Check sheet for the modelled part. Datum: model origin and axes. Units: mm. Give positions to 0.01 mm unless a question says otherwise; leave off trailing zeros. Loops run counter-clockwise (first coordinate to the right, second up) from the corner with the lowest first, then second, coordinate; pieces in that order, holes last. Notation, with made-up numbers: (10, 80.25) - (43, 80.25) arc R8 cw to (43, 93.25) - close; hole circle Ø3 at (74.25, 38). An arc over 180 degrees is marked (long way). Use CSV: the item, a comma, the result in double quotes.
Autodesk Inventor part; units mm, degrees
ref_plane "MidSidePlane" through (0, 0, 10) normal (0, 0, 1) x (1, 0, 0)
ref_plane "YZ Plane" through (0, 0, 0) normal (1, 0, 0) x (0, 1, 0)
ref_plane "XZ Plane" through (0, 0, 0) normal (0, 1, 0) x (-1, 0, 0)
sketch "ShaftProfile" plane through (0, 0, 0) normal (0, 0, 1) x (1, 0, 0)
  line L0 (-64, 0) -> (118, 0) construction
  line L1 (-38, 9) -> (92, 9)
  line L2 (92, 9) -> (92, 0)
  line L3 (-38, 0) -> (-38, 9)
  line L4 (-38, 0) -> (92, 0)
  point P0 (0, 0)
  dimension "d1" = 130
  dimension "d2" = 9
  dimension "d4" = 38
revolve "ShaftFeature" add sketch "ShaftProfile" angle 360 about axis through (-38, 0, 0) along (1, 0, 0)
sketch "Sketch2" plane through (-38, 0, 0) normal (-1, 0, 0) x (0, 0, 1)
  circle A0 centre (0, 0) radius 9
hole "ShaftHoleFeature" at (-38, 0, 0) direction (1, 0, 0) diameter 16 end through all
ref_plane "MidSidePlane" through (0, 0, 10) normal (0, 0, 1) x (1, 0, 0)
sketch "CapHoles" plane through (0, 0, 10) normal (0, 0, 1) x (1, 0, 0)
  line L0 (92, -9) -> (92, 9) construction
  line L1 (-38, -9) -> (-38, 9) construction
  line L2 (-45, 0) -> (4, 0) construction
  circle A0 centre (-33.5, 0) radius 1.25
  circle A1 centre (87.5, 0) radius 1.25
  dimension "d24" = 2.5
  dimension "d25" = 4.5
  dimension "d26" = 4.5
extrude "CapHolesFeature" cut sketch "CapHoles" against normal through all
equation "\"d26\" = d25"
properties part number "BackPair1PistonShaft"
1. Sectioned sample at D-D, the plane x = 62. Record the boundary of the cut face in (y, z).
Completed:
outline,"circle Ø18 at (0, 0); hole circle Ø16 at (0, 0)"
2. Release check for a two-part mould opening along Y. For faces 1 (the face through (86.25, 0.05, 8.46)), 2 (the face through (27.91, -1.172, 8.923)), 3 (the face through (27.91, 7.81, -1.73)) record: released by +Y, released by -Y, zero draft, split by the parting line, or undercut.
Completed:
face 1,"undercut"
face 2,"split by the parting line"
face 3,"undercut"
3. Scan lines: line 1 along X through (y, z) = (0, -8.3); line 2 along Z through (x, y) = (44.5, 0); line 3 along Y through (x, z) = (-28, -0.5). Record each from-to range of solid material in increasing order.
Completed:
line 1,"x = -38 to -34.75, -32.25 to 86.25, 88.75 to 92"
line 2,"z = -9 to -8, 8 to 9"
line 3,"y = -8.99 to -7.98, 7.98 to 8.99"
4. Go/stop test with a flat-tipped pin: pin 1 Ø10 at (x, y) = (15.5, -6.5) entering from +Z. Record where the tip stops, or that it passes through.
Completed:
pin 1,"stops at z = 8.87"
5. Sectioned sample at C-C, the plane z = 5.5. Record the boundary of the cut face in (x, y), and give its area (3 significant figures).
Completed:
outline,"(-38, -7.12) - (92, -7.12) - (92, -5.81) - (-38, -5.81) - close; (-38, 5.81) - (92, 5.81) - (92, 7.12) - (-38, 7.12) - close"
area,"342 mm²"
6. Sectioned sample at A-A, the plane y = 0. Record the boundary of the cut face in (x, z).
Completed:
outline,"(-38, -9) - (-34.75, -9) - (-34.75, -8) - (-38, -8) - close; (-38, 8) - (-34.75, 8) - (-34.75, 9) - (-38, 9) - close; (-32.25, -9) - (86.25, -9) - (86.25, -8) - (-32.25, -8) - close; (-32.25, 8) - (86.25, 8) - (86.25, 9) - (-32.25, 9) - close; (88.75, -9) - (92, -9) - (92, -8) - (88.75, -8) - close; (88.75, 8) - (92, 8) - (92, 9) - (88.75, 9) - close"
7. Sectioned sample at B-B, the plane x = 87.5. Record the boundary of the cut face in (y, z).
Completed:
outline,"(-1.25, -8.91) - (-1.25, -7.9) arc R8 cw to (-1.25, 7.9) - (-1.25, 8.91) arc R9 ccw to start; (1.25, -8.91) arc R9 ccw to (1.25, 8.91) - (1.25, 7.9) arc R8 cw to (1.25, -7.9) - close"
